Verification items for the finished model (mm, model axes). Round coordinates to 2 decimals unless told otherwise and drop trailing zeros. Loops run counter-clockwise (first coordinate to the right, second up) from the corner with the lowest first, then second, coordinate; pieces in that order, holes last. Notation, with made-up numbers: M 84.25,2.25 L 131.25,2.25 A20 cw 131.25,21.25 Z; hole C -34.5,-29.75 d10. An arc over 180 degrees is marked long. Answer as CSV lines item,"result".
```python
from build123d import *

# Parameters (mm, degrees)
F1_DEPTH = 10


# Not quite as in the source:
# - a feature names something its author has since deleted; it is built from what else it names


with BuildPart() as f1:
    # F0 (on Front) → F1 (new body)
    with BuildSketch(Plane.XZ):
        with BuildLine():
            add(Edge.make_bspline(
                [(10, 0), (8.6317372981, 1.0499048978), (8.645995668, 3.0249524489), (8.6602540378, 5)],
                knots=[0.6299429387, 0.6299429387, 0.6299429387, 0.6299429387, 1, 1, 1, 1], degree=3))
            ThreePointArc((10, 0), (9.6592582629, 2.588190451), (8.6602540378, 5))
        make_face()
        with BuildLine():
            add(Edge.make_bspline(
                [(25, 0), (18.6645871914, -0.8936191818), (12.3291743827, -1.7872383636), (10, 0)],
                knots=[0, 0, 0, 0, 0.6299429387, 0.6299429387, 0.6299429387, 0.6299429387], degree=3))
            ThreePointArc((10, 0), (9.6592582629, -2.588190451), (8.6602540378, -5))
            Line((8.6602540378, -5), (25, 0))
        make_face()
        with BuildLine():
            ThreePointArc((8.6602540378, -5), (9.6592582629, -2.588190451), (10, 0))
            Line((10, 0), (5, 0))
            Line((5, 0), (5, -4.9574967987))
            Line((5, -4.9574967987), (5, -5))
            Line((5, -5), (8.6602540378, -5))
        make_face()
        with BuildLine():
            Line((5, 0), (10, 0))
            add(Edge.make_bspline(
                [(10, 0), (8.6317372981, 1.0499048978), (8.645995668, 3.0249524489), (8.6602540378, 5)],
                knots=[0.6299429387, 0.6299429387, 0.6299429387, 0.6299429387, 1, 1, 1, 1], degree=3))
            Line((8.6602540378, 5), (5, 5))
            Line((5, 5), (5, 0))
        make_face()
        with BuildLine():
            Line((5, 5), (8.6602540378, 5))
            ThreePointArc((8.6602540378, 5), (7.0710678119, 7.0710678119), (5, 8.6602540378))
            Line((5, 8.6602540378), (5, 5))
        make_face()
        with BuildLine():
            ThreePointArc((5, -8.6602540378), (7.0710678119, -7.0710678119), (8.6602540378, -5))
            Line((8.6602540378, -5), (5, -5))
            Line((5, -5), (5, -8.6602540378))
        make_face()
        with BuildLine():
            ThreePointArc((0, 5), (3.5355339059, 3.5355339059), (5, 0))
            Line((5, 0), (5, 5))
            Line((5, 5), (4.9574967987, 5))
            Line((4.9574967987, 5), (0, 5))
        make_face()
        with BuildLine():
            Line((5, -4.9574967987), (5, 0))
            ThreePointArc((5, 0), (3.5355339059, -3.5355339059), (0, -5))
            Line((0, -5), (4.9574967987, -5))
            Line((4.9574967987, -5), (5, -5))
            Line((5, -5), (5, -4.9574967987))
        make_face()
        with BuildLine():
            Line((5, 5), (5, 8.6602540378))
            ThreePointArc((5, 8.6602540378), (2.588190451, 9.6592582629), (0, 10))
            Line((0, 10), (0, 5))
            Line((0, 5), (4.9574967987, 5))
            Line((4.9574967987, 5), (5, 5))
        make_face()
        with BuildLine():
            ThreePointArc((0, 10), (2.588190451, 9.6592582629), (5, 8.6602540378))
            Line((5, 8.6602540378), (0, 25))
            add(Edge.make_bspline(
                [(0, 25), (0.8936191818, 18.6645871914), (1.7872383636, 12.3291743827), (0, 10)],
                knots=[0, 0, 0, 0, 0.6299429387, 0.6299429387, 0.6299429387, 0.6299429387], degree=3))
        make_face()
        with BuildLine():
            add(Edge.make_bspline(
                [(0, -10), (1.0499048978, -8.6317372981), (3.0249524489, -8.645995668), (5, -8.6602540378)],
                knots=[0.6299429387, 0.6299429387, 0.6299429387, 0.6299429387, 1, 1, 1, 1], degree=3))
            Line((5, -8.6602540378), (5, -5))
            Line((5, -5), (4.9574967987, -5))
            Line((4.9574967987, -5), (0, -5))
            Line((0, -5), (0, -10))
        make_face()
        with BuildLine():
            ThreePointArc((0, -10), (2.588190451, -9.6592582629), (5, -8.6602540378))
            add(Edge.make_bspline(
                [(0, -10), (1.0499048978, -8.6317372981), (3.0249524489, -8.645995668), (5, -8.6602540378)],
                knots=[0.6299429387, 0.6299429387, 0.6299429387, 0.6299429387, 1, 1, 1, 1], degree=3))
        make_face()
        with BuildLine():
            Line((-5, 5), (0, 5))
            Line((0, 5), (0, 10))
            add(Edge.make_bspline(
                [(0, 10), (-1.0499048978, 8.6317372981), (-3.0249524489, 8.645995668), (-5, 8.6602540378)],
                knots=[0.6299429387, 0.6299429387, 0.6299429387, 0.6299429387, 1, 1, 1, 1], degree=3))
            Line((-5, 8.6602540378), (-5, 5))
        make_face()
        with BuildLine():
            ThreePointArc((-5, 0), (-3.5355339059, 3.5355339059), (0, 5))
            Line((0, 5), (-5, 5))
            Line((-5, 5), (-5, 0))
        make_face()
        with BuildLine():
            Line((0, -10), (0, -5))
            Line((0, -5), (-5, -5))
            Line((-5, -5), (-5, -8.6602540378))
            ThreePointArc((-5, -8.6602540378), (-2.588190451, -9.6592582629), (0, -10))
        make_face()
        with BuildLine():
            Line((-5, -5), (0, -5))
            ThreePointArc((0, -5), (-3.5355339059, -3.5355339059), (-5, 0))
            Line((-5, 0), (-5, -4.9574967987))
            Line((-5, -4.9574967987), (-5, -5))
        make_face()
        with BuildLine():
            add(Edge.make_bspline(
                [(0, 10), (-1.0499048978, 8.6317372981), (-3.0249524489, 8.645995668), (-5, 8.6602540378)],
                knots=[0.6299429387, 0.6299429387, 0.6299429387, 0.6299429387, 1, 1, 1, 1], degree=3))
            ThreePointArc((0, 10), (-2.588190451, 9.6592582629), (-5, 8.6602540378))
        make_face()
        with BuildLine():
            add(Edge.make_bspline(
                [(0, -25), (-0.8936191818, -18.6645871914), (-1.7872383636, -12.3291743827), (0, -10)],
                knots=[0, 0, 0, 0, 0.6299429387, 0.6299429387, 0.6299429387, 0.6299429387], degree=3))
            ThreePointArc((0, -10), (-2.588190451, -9.6592582629), (-5, -8.6602540378))
            Line((-5, -8.6602540378), (0, -25))
        make_face()
        with BuildLine():
            Line((-5, -4.9574967987), (-5, 0))
            Line((-5, 0), (-10, 0))
            add(Edge.make_bspline(
                [(-10, 0), (-8.6317383367, -1.0514075248), (-8.6459961873, -3.0257037624), (-8.6602540378, -5)],
                knots=[0.6299429387, 0.6299429387, 0.6299429387, 0.6299429387, 1, 1, 1, 1], degree=3))
            Line((-8.6602540378, -5), (-5, -5))
            Line((-5, -5), (-5, -4.9574967987))
        make_face()
        with BuildLine():
            Line((-10, 0), (-5, 0))
            Line((-5, 0), (-5, 5))
            Line((-5, 5), (-8.6602540378, 5))
            ThreePointArc((-8.6602540378, 5), (-9.6592582629, 2.588190451), (-10, 0))
        make_face()
        with BuildLine():
            Line((-8.6602540378, 5), (-5, 5))
            Line((-5, 5), (-5, 8.6602540378))
            ThreePointArc((-5, 8.6602540378), (-7.0710678119, 7.0710678119), (-8.6602540378, 5))
        make_face()
        with BuildLine():
            Line((-5, -8.6602540378), (-5, -5))
            Line((-5, -5), (-8.6602540378, -5))
            ThreePointArc((-8.6602540378, -5), (-7.0710678119, -7.0710678119), (-5, -8.6602540378))
        make_face()
        with BuildLine():
            add(Edge.make_bspline(
                [(-24.9999856665, 0.0207365385), (-18.6645791406, 0.9052664015), (-12.3291726147, 1.7897962644), (-10, 0)],
                knots=[0, 0, 0, 0, 0.6299429387, 0.6299429387, 0.6299429387, 0.6299429387], degree=3))
            ThreePointArc((-10, 0), (-9.6592582629, 2.588190451), (-8.6602540378, 5))
            Line((-8.6602540378, 5), (-24.9999856665, 0.0207365385))
        make_face()
        with BuildLine():
            add(Edge.make_bspline(
                [(-10, 0), (-8.6317383367, -1.0514075248), (-8.6459961873, -3.0257037624), (-8.6602540378, -5)],
                knots=[0.6299429387, 0.6299429387, 0.6299429387, 0.6299429387, 1, 1, 1, 1], degree=3))
            ThreePointArc((-10, 0), (-9.6592582629, -2.588190451), (-8.6602540378, -5))
        make_face()
    extrude(amount=F1_DEPTH)


solid = f1.part
```
1) Section check C-C (x = 7). Record the cut outline in (y, z).
Here are the results:
outline,"M -10,-7.14 L 0,-7.14 L 0,7.14 L -10,7.14 Z"
2) Section check A-A (x = -4). Record the cut outline in (y, z).
Here are the results:
outline,"M -10,-11.93 L 0,-11.93 L 0,-3 L -10,-3 Z; M -10,3 L 0,3 L 0,9.17 L -10,9.17 Z"
3) Material ranges on probe 1 along X at (y, z) = (-2, -5.5); probe 2 along Z at (x, y) = (15, -2.25); probe 3 along X at (y, z) = (-4, 19.5), recorded low to high.
Here are the results:
probe 1,"x = -8.35 to 8.35"
probe 2,"z = -3.06 to -1.03"
probe 3,"x = 0.72 to 1.68"
4) Section check B-B (z = -3). Record the cut outline in (x, y).
Here are the results:
outline,"M -9.54,-10 L -4,-10 L -4,0 L -9.54,0 Z; M 4,-10 L 15.2,-10 L 15.2,0 L 4,0 Z"
5) Go/stop test with flat-tipped pins: pin 1 (1.5 mm diameter, centred on x = -1.5, z = 14.5, fed in from -Y) (1 decimal); pin 2 (4 mm diameter, centred on y = -8, z = 9.5, fed in from +X); pin 3 (4 mm diameter, centred on x = -10.5, y = -6.5, fed in from -Z). Record where each tip stops, or that it passes through.
Here are the results:
pin 1,"passes through"
pin 2,"stops at x = 6.61"
pin 3,"stops at z = -5.27"
